Verification items for this drawing (mm, ordinates from the low corner). Give positions to 0.01 mm unless a question says otherwise; leave off trailing zeros. Write each loop counter-clockwise with the first axis right and the second up, starting at its lowest first coordinate (ties: lowest second). Pieces come first, ordered by that corner, then holes. Notation, with made-up numbers: (6.25, 79) -> (21.25, 79) arc R34 ccw to (21.25, 113) -> close; hole circle Ø8 at (-3.5, -11.75). An arc over 180 degrees is marked (long way). Answer as a JSON object with one key per item and string values.
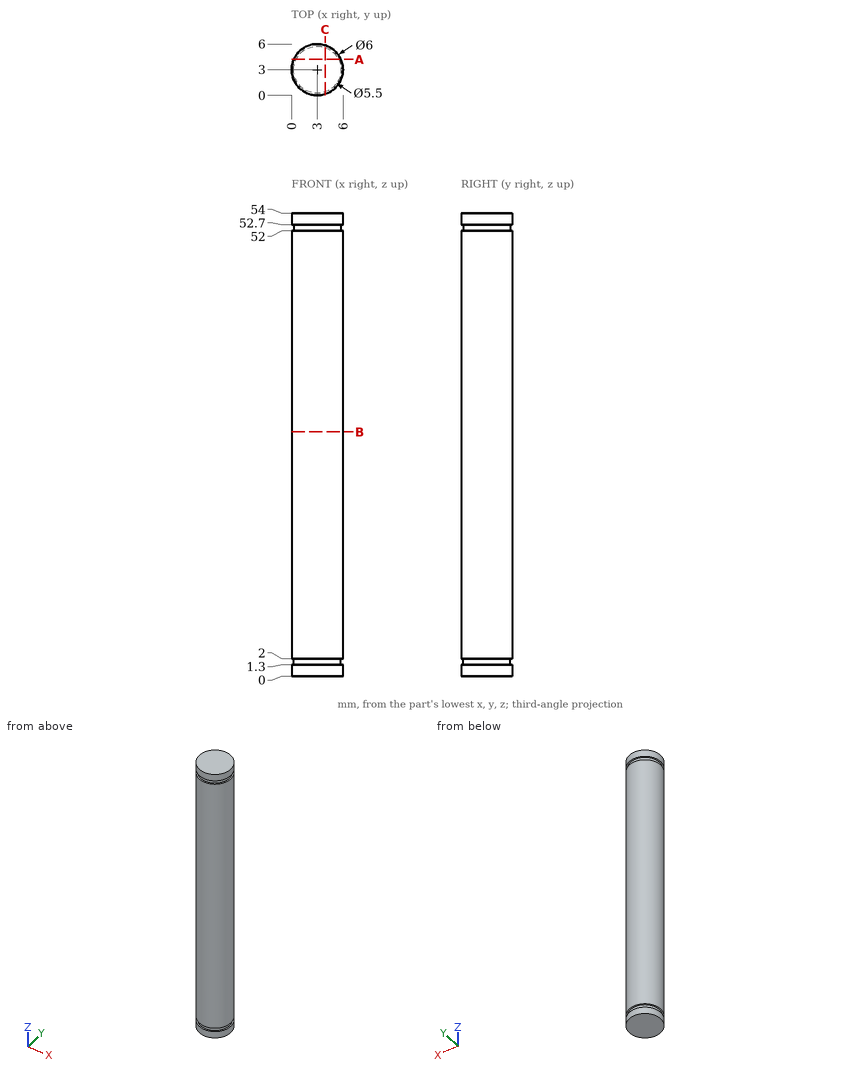
1. Scan lines: L1, parallel to Y at x = 3.1, z = 43.5; L2, parallel to Y at x = 2.4, z = 32; L3, parallel to X at y = 5.6, z = 22. Record each from-to range of solid material in increasing order. Write a range as [from, to].
Determined:
{"L1": "[0, 6]", "L2": "[0.06, 5.94]", "L3": "[1.5, 4.5]"}
2. Sectioned sample at C-C, the plane x = 3.9. Enter the section's corners in (y, z).
Determined:
{"outline": "(0.14, 0) -> (5.86, 0) -> (5.86, 1.3) -> (5.6, 1.3) -> (5.6, 2) -> (5.86, 2) -> (5.86, 52) -> (5.6, 52) -> (5.6, 52.7) -> (5.86, 52.7) -> (5.86, 54) -> (0.14, 54) -> (0.14, 52.7) -> (0.4, 52.7) -> (0.4, 52) -> (0.14, 52) -> (0.14, 2) -> (0.4, 2) -> (0.4, 1.3) -> (0.14, 1.3) -> close"}
3. Go/stop test with a flat-tipped pin: P1, Ø1.5, axis at x = 2, z = 23.5, coming from the -Y side. Record where the tip stops, or that it passes through.
Determined:
{"P1": "y = 0.01"}
4. Sectioned sample at B-B, the plane z = 28.5. Enter the section's corners in (x, y), plus the area to 3 significant figures.
Determined:
{"outline": "circle Ø6 at (3, 3)", "area": "28.3 mm^2"}
5. Sectioned sample at A-A, the plane y = 4.2. Enter the section's corners in (x, z), plus the area to 3 significant figures.
Determined:
{"outline": "(0.25, 0) -> (5.75, 0) -> (5.75, 1.3) -> (5.47, 1.3) -> (5.47, 2) -> (5.75, 2) -> (5.75, 52) -> (5.47, 52) -> (5.47, 52.7) -> (5.75, 52.7) -> (5.75, 54) -> (0.25, 54) -> (0.25, 52.7) -> (0.53, 52.7) -> (0.53, 52) -> (0.25, 52) -> (0.25, 2) -> (0.53, 2) -> (0.53, 1.3) -> (0.25, 1.3) -> close", "area": "296 mm^2"}
